Verification items for the finished model (mm, model axes). Face numbers are marked on the shaded views. Round coordinates to 2 decimals unless told otherwise and drop trailing zeros. Loops run counter-clockwise (first coordinate to the right, second up) from the corner with the lowest first, then second, coordinate; pieces in that order, holes last. Notation, with made-up numbers: (-35.75, -32.75) - (19.25, -32.75) arc R30 cw to (19.25, -4.75) - close; hole circle Ø2 at (61, -8). An arc over 180 degrees is marked (long way). Use a Markdown table: item, result. Add a question column.
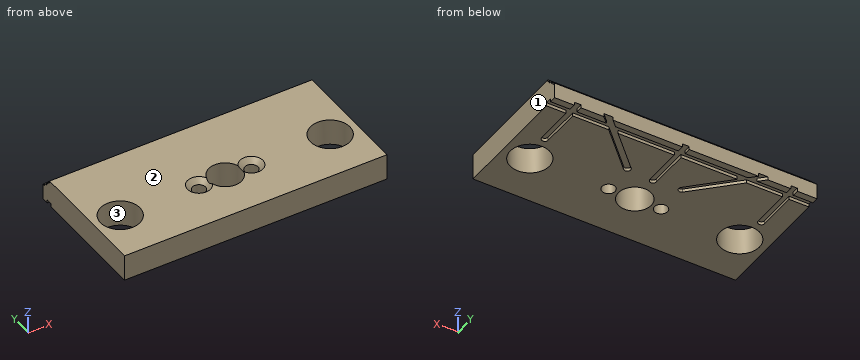
```python
from build123d import *

# Parameters (mm, degrees)
SKETCH_1_W                     = 80
SKETCH_1_H                     = 60
EXTRUDE_1_DEPTH                = 8
HOLE_WIZARD_12_0_12_1_D        = 12
HOLE_WIZARD_10_0_10_2_D        = 10
HOLE_WIZARD_M3_5_1_D           = 4
HOLE_WIZARD_M3_5_1_CSINK_D     = 7
HOLE_WIZARD_M3_5_1_CSINK_ANGLE = 90
CUT_EXTRUDE_1_DEPTH            = 1
CUT_EXTRUDE_2_REACH            = 95.053
CUT_EXTRUDE_3_REACH            = 94.961
SKETCH_29_W                    = 80
SKETCH_29_H                    = 20


with BuildPart() as part:
    # 草图1 → 凸台-拉伸1 (new body)
    with BuildSketch(Plane(origin=(0, 0, 1), x_dir=(-1, 0, 0), z_dir=(0, 0, -1))):
        with Locations((-40, 16.666666667)):
            Rectangle(SKETCH_1_W, SKETCH_1_H)
    extrude(amount=-EXTRUDE_1_DEPTH)

    # Ø12.0 (12) 直径孔1 (through all)
    with Locations(Plane.XY.offset(9)):
        with Locations((72, 21.666666667), (8, 21.666666667)):
            Hole(HOLE_WIZARD_12_0_12_1_D / 2)

    # Ø10.0 (10) 直径孔2 (through all)
    with Locations(Plane(origin=(0, 0, 1), x_dir=(-1, 0, 0), z_dir=(0, 0, -1))):
        with Locations((-40, 21.666666667)):
            Hole(HOLE_WIZARD_10_0_10_2_D / 2)

    # M3.5 平头机械螺钉的锥形沉头孔1 (through all)
    with Locations(Plane.XY.offset(9)):
        with Locations((32, 21.666666667), (48, 21.666666667)):
            CounterSinkHole(HOLE_WIZARD_M3_5_1_D / 2, HOLE_WIZARD_M3_5_1_CSINK_D / 2, counter_sink_angle=HOLE_WIZARD_M3_5_1_CSINK_ANGLE)

    # 草图27 → 切除-拉伸1 (cut)
    with BuildSketch(Plane(origin=(0, 0, 1), x_dir=(-1, 0, 0), z_dir=(0, 0, -1))):
        with BuildLine():
            ThreePointArc((-41, 30.666666667), (-40, 29.666666667), (-39, 30.666666667))
            Line((-39, 30.666666667), (-39, 42.666666667))
            Line((-39, 42.666666667), (-21.828427125, 42.666666667))
            Line((-21.828427125, 42.666666667), (-32.414213562, 32.080880229))
            ThreePointArc((-32.414213562, 32.080880229), (-32.414213562, 30.666666667), (-31, 30.666666667))
            Line((-31, 30.666666667), (-19, 42.666666667))
            Line((-19, 42.666666667), (-8, 42.666666667))
            Line((-8, 42.666666667), (-8, 30.666666667))
            ThreePointArc((-8, 30.666666667), (-7, 29.666666667), (-6, 30.666666667))
            Line((-6, 30.666666667), (-6, 42.666666667))
            Line((-6, 42.666666667), (0, 42.666666667))
            Line((0, 42.666666667), (0, 44.666666667))
            Line((0, 44.666666667), (-6, 44.666666667))
            Line((-6, 44.666666667), (-6, 46.666666667))
            Line((-6, 46.666666667), (-8, 46.666666667))
            Line((-8, 46.666666667), (-8, 44.666666667))
            Line((-8, 44.666666667), (-17, 44.666666667))
            Line((-17, 44.666666667), (-15, 46.666666667))
            Line((-15, 46.666666667), (-16.414213562, 48.080880229))
            Line((-16.414213562, 48.080880229), (-19.828427125, 44.666666667))
            Line((-19.828427125, 44.666666667), (-39, 44.666666667))
            Line((-39, 44.666666667), (-39, 46.666666667))
            Line((-39, 46.666666667), (-41, 46.666666667))
            Line((-41, 46.666666667), (-41, 44.666666667))
            Line((-41, 44.666666667), (-60.171572875, 44.666666667))
            Line((-60.171572875, 44.666666667), (-63.585786438, 48.080880229))
            Line((-63.585786438, 48.080880229), (-65, 46.666666667))
            Line((-65, 46.666666667), (-63, 44.666666667))
            Line((-63, 44.666666667), (-72, 44.666666667))
            Line((-72, 44.666666667), (-72, 46.666666667))
            Line((-72, 46.666666667), (-74, 46.666666667))
            Line((-74, 46.666666667), (-74, 44.666666667))
            Line((-74, 44.666666667), (-80, 44.666666667))
            Line((-80, 44.666666667), (-80, 42.666666667))
            Line((-80, 42.666666667), (-74, 42.666666667))
            Line((-74, 42.666666667), (-74, 30.666666667))
            ThreePointArc((-74, 30.666666667), (-73, 29.666666667), (-72, 30.666666667))
            Line((-72, 30.666666667), (-72, 42.666666667))
            Line((-72, 42.666666667), (-61, 42.666666667))
            Line((-61, 42.666666667), (-49, 30.666666667))
            ThreePointArc((-49, 30.666666667), (-47.585786438, 30.666666667), (-47.585786438, 32.080880229))
            Line((-47.585786438, 32.080880229), (-58.171572875, 42.666666667))
            Line((-58.171572875, 42.666666667), (-41, 42.666666667))
            Line((-41, 42.666666667), (-41, 30.666666667))
        make_face()
    extrude(amount=-CUT_EXTRUDE_1_DEPTH, mode=Mode.SUBTRACT)

    # 草图28 → 切除-拉伸2 (cut, up to next)
    with BuildSketch(Plane.ZY, mode=Mode.PRIVATE) as cut_extrude_2_sk1:
        Polygon((9, 46.666666667), (5.8, 46.666666667), (5.8, 45.866666667), (6.6, 45.866666667), (6.6, 45.066666667), (7.4, 45.066666667), (7.4, 44.266666667), (8.2, 44.266666667), (8.2, 43.466666667), (9, 43.466666667), align=None)
    cut_extrude_2_tool1 = extrude(cut_extrude_2_sk1.sketch, amount=-CUT_EXTRUDE_2_REACH, mode=Mode.PRIVATE) & part.part
    add(cut_extrude_2_tool1.solids().sort_by_distance((0, 45.466667, 7.8))[0], mode=Mode.SUBTRACT)

    # 草图29 → 切除-拉伸3 (cut, up to next)
    with BuildSketch(Plane(origin=(0, 0, 1), x_dir=(-1, 0, 0), z_dir=(0, 0, -1)), mode=Mode.PRIVATE) as cut_extrude_3_sk1:
        with Locations((-40, -3.333333333)):
            Rectangle(SKETCH_29_W, SKETCH_29_H)
    cut_extrude_3_tool1 = extrude(cut_extrude_3_sk1.sketch, amount=-CUT_EXTRUDE_3_REACH, mode=Mode.PRIVATE) & part.part
    add(cut_extrude_3_tool1.solids().sort_by_distance((40, -3.333333, 1))[0], mode=Mode.SUBTRACT)


solid = part.part
```
Q1. Go/stop test with flat-tipped pins: pin 1 Ø0.6 at (x, z) = (48.5, 8) entering from +Y; pin 2 Ø0.9 at (x, y) = (27, 45) entering from +Z. Record where each tip stops, or that it passes through.
Q2. Section check B-B on x = 16. Record the cut outline in (y, z), plus the area to 3 significant figures.
Q3. Section check C-C on z = 3.25. Record the cut outline in (x, y).
Q4. Thickness scan on line 1 along Y through (x, z) = (40, 6.5); line 2 along Y through (x, z) = (32, 3.75); line 3 along X through (y, z) = (24, 4.75). Record the ranges inside material, lowest first.
Q5. Section check A-A on x = 40. Record the cut outline in (y, z).
Q6. Section check D-D on x = 7. Record the cut outline in (y, z).
Q7. Release check for a two-part mould opening along X. For the marked faces 1, 2 and 3 record: +X half, -X half, draft (parallel to the pull), parting line (faces both ways), or undercut.
Determined:
| question | item | result |
|---|---|---|
| 1 | pin 1 | stops at y = 44.27 |
| 1 | pin 2 | stops at z = 7.4 |
| 2 | outline | (6.67, 1) - (42.67, 1) - (42.67, 2) - (44.67, 2) - (44.67, 1) - (45.67, 1) - (45.67, 2) - (46.67, 2) - (46.67, 5.8) - (45.87, 5.8) - (45.87, 6.6) - (45.07, 6.6) - (45.07, 7.4) - (44.27, 7.4) - (44.27, 8.2) - (43.47, 8.2) - (43.47, 9) - (6.67, 9) - close |
| 2 | area | 311 mm² |
| 3 | outline | (0, 6.67) - (80, 6.67) - (80, 46.67) - (0, 46.67) - close; hole circle Ø12 at (8, 21.67); hole circle Ø4 at (32, 21.67); hole circle Ø10 at (40, 21.67); hole circle Ø4 at (48, 21.67); hole circle Ø12 at (72, 21.67) |
| 4 | line 1 | y = 6.67 to 16.67, 26.67 to 45.87 |
| 4 | line 2 | y = 6.67 to 19.67, 23.67 to 46.67 |
| 4 | line 3 | x = 0 to 2.47, 13.53 to 35.58, 44.42 to 66.47, 77.53 to 80 |
| 5 | outline | (6.67, 1) - (16.67, 1) - (16.67, 9) - (6.67, 9) - close; (26.67, 1) - (29.67, 1) - (29.67, 2) - (46.67, 2) - (46.67, 5.8) - (45.87, 5.8) - (45.87, 6.6) - (45.07, 6.6) - (45.07, 7.4) - (44.27, 7.4) - (44.27, 8.2) - (43.47, 8.2) - (43.47, 9) - (26.67, 9) - close |
| 6 | outline | (6.67, 1) - (15.75, 1) - (15.75, 9) - (6.67, 9) - close; (27.58, 1) - (29.67, 1) - (29.67, 2) - (46.67, 2) - (46.67, 5.8) - (45.87, 5.8) - (45.87, 6.6) - (45.07, 6.6) - (45.07, 7.4) - (44.27, 7.4) - (44.27, 8.2) - (43.47, 8.2) - (43.47, 9) - (27.58, 9) - close |
| 7 | face 1 | +X half |
| 7 | face 2 | draft |
| 7 | face 3 | undercut |
